Work out the finished part from the listing and answer in its coordinate system (mm). Face numbers are marked on the shaded views. A direction names the side the tool comes from. Coordinates: 2 decimals unless noted, no trailing zeros. Order: outer loops, then holes, each group sorted by start corner. A loop starts at its lowest first (then second) coordinate and runs counter-clockwise, first axis right, second up. Notation, with made-up numbers: M -8.75,14 L 42.25,14 A29 cw 42.25,49 Z; hole C 57,85 d6. An arc over 180 degrees is marked long. Use a Markdown table: item, result.
from build123d import *

# Parameters (mm, degrees)
EXTRUDE_1_DEPTH     = 80
SKETCH_4_R          = 7.5
CUT_EXTRUDE_1_DEPTH = 119.184803146


with BuildPart() as part:
    # 草图3 → 凸台-拉伸1 (new body)
    with BuildSketch(Plane.XY):
        with BuildLine():
            Line((60.702784473, 47), (-27.297215527, 47))
            Line((-27.297215527, 47), (-27.297215527, 24))
            Line((-27.297215527, 24), (-39.797215527, 24))
            Line((-39.797215527, 24), (-39.797215527, 0))
            Line((-39.797215527, 0), (-19.797215527, 0))
            add(Edge.make_bspline(
                [(-19.797215527, 0), (16.702784473, 32), (53.202784473, 0)],
                knots=[0, 0, 0, 1, 1, 1], degree=2))
            Line((53.202784473, 0), (73.202784473, 0))
            Line((73.202784473, 0), (73.202784473, 24))
            Line((73.202784473, 24), (60.702784473, 24))
            Line((60.702784473, 24), (60.702784473, 47))
        make_face()
    extrude(amount=EXTRUDE_1_DEPTH)

    # 草图4 → 切除-拉伸1 (cut, through all)
    with BuildSketch(Plane(origin=(0, 47, 0), x_dir=(1, 0, 0), z_dir=(0, 1, 0))):
        with Locations(Location((20.202784473, -40, 0), (0, 0, 180))):
            Circle(SKETCH_4_R)
    extrude(amount=-CUT_EXTRUDE_1_DEPTH, mode=Mode.SUBTRACT)


solid = part.part
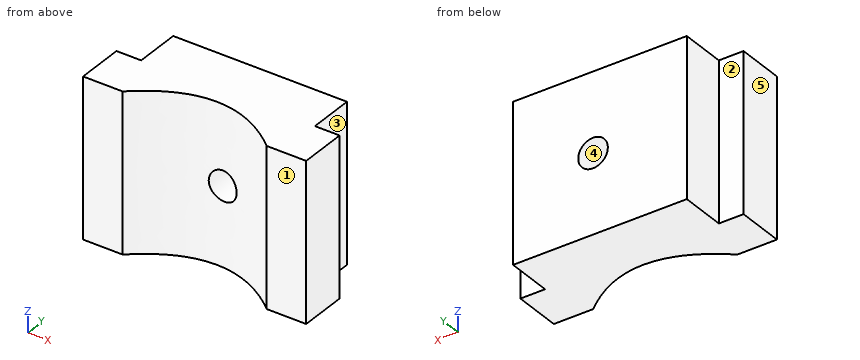
(1) Which of the six approach directions +Z, -Z, +X, -X, +Y, -Y give full straight-line access (tool end or side, diameter ignored) to the marked faces 1 and 2?
Conclusion:
| item | result |
|---|---|
| face 1 | +Z, -Z, +X, -X, -Y |
| face 2 | +Z, -Z, -X, +Y |
(2) Determine the mould class of the marked faces 3, 4 and 5 for opening direction X: pulls with the +X half, pulls with the -X half, needs draft (parallel to the pull), parting line crosses it, or undercut.
Conclusion:
| item | result |
|---|---|
| face 3 | pulls with the +X half |
| face 4 | undercut |
| face 5 | pulls with the -X half |
(3) Straight lines are drawn through the part: L1, parallel to X at y = 24.5, z = 40; L2, parallel to X at y = 23, z = 40.5; L3, parallel to Y at x = -31, z = 24.5. For each, find the intervals that lie inside material, in ascending order.
Conclusion:
| item | result |
|---|---|
| L1 | -27.3 to 12.7, 27.7 to 60.7 |
| L2 | -39.8 to 12.72, 27.69 to 73.2 |
| L3 | 0 to 24 |
(4) A cutting plane is placed at A-A (y = 39.5). Determine the outline of the cut face in (x, z).
Conclusion:
| item | result |
|---|---|
| outline | M -27.3,0 L 60.7,0 L 60.7,80 L -27.3,80 Z; hole C 20.2,40 d15 |
(5) Given P1, Ø19.5, axis at x = 20.2, z = 40, coming from the -Y side; P2, Ø1.5, axis at x = 48.5, z = 64, coming from the -Y side; P3, Ø7, axis at y = 41, z = 44, coming from the -X side, each flat-ended and moving along its own axis, determine where each tip first touches the part or whether it passes through.
Conclusion:
| item | result |
|---|---|
| P1 | y = 13.89 |
| P2 | y = 3.28 |
| P3 | x = -27.3 |
